Source: CAD feature listing. Evaluate the final solid. Frame: model axes, mm. A direction names the side the tool comes from. Give positions to 0.01 mm unless a question says otherwise; leave off trailing zeros. Order: outer loops, then holes, each group sorted by start corner. A loop starts at its lowest first (then second) coordinate and runs counter-clockwise, first axis right, second up. Notation, with made-up numbers: (52.25, 14.5) -> (92.25, 14.5) arc R12 ccw to (92.25, 25.5) -> close; hole circle Ø3 at (-29, 55). An arc over 180 degrees is marked (long way). Use CSV: the item, a comma, the result in double quotes.
```python
from build123d import *

# Parameters (mm, degrees)
F1_DEPTH = 2.286
F2_DEPTH = 0.254
F3_W     = 12.7
F3_H     = 1.016
F4_DEPTH = 0.254


with BuildPart() as f1:
    # F0 (on Top) → F1 (new body)
    with BuildSketch(Plane.XY):
        with BuildLine():
            Line((-13.1568801942, -7.1914618043), (-15.685681705, -13.4825458221))
            add(Edge.make_bspline(
                [(-15.685681705, -13.4825458221), (-13.2321975411, -12.2693498698), (-11.0318471059, -10.4379374373), (-8.9577929719, -8.5581073527)],
                knots=[0, 0, 0, 0, 6.5648699385, 6.5648699385, 6.5648699385, 6.5648699385], degree=3))
            add(Edge.make_bspline(
                [(-8.9577929719, -8.5581073527), (-2.326521087, -2.5478185256), (3.0136976356, 3.9574156183), (11.2083703228, -7.6654970922)],
                knots=[6.5648699385, 6.5648699385, 6.5648699385, 6.5648699385, 27.554407645, 27.554407645, 27.554407645, 27.554407645], degree=3))
            add(Edge.make_bspline(
                [(11.2083703228, -7.6654970922), (12.3264260334, -9.2512912326), (13.497617481, -11.1745413121), (14.7324733271, -13.4825458221)],
                knots=[27.554407645, 27.554407645, 27.554407645, 27.554407645, 30.4181550321, 30.4181550321, 30.4181550321, 30.4181550321], degree=3))
            Line((14.7324733271, -13.4825458221), (12.2638968299, -7.2552273315))
            Line((12.2638968299, -7.2552273315), (5.6394149783, 9.4559251776))
            Line((5.6394149783, 9.4559251776), (-0.3707793305, 24.6174541779))
            Line((-0.3707793305, 24.6174541779), (-6.4710147318, 9.441453502))
            Line((-6.4710147318, 9.441453502), (-13.1568801942, -7.1914618043))
        make_face()
        with BuildLine():
            add(Edge.make_bspline(
                [(-6.4710147318, 9.441453502), (-39.6247541981, 4.06906696), (-13.1568801942, -7.1914618043)],
                knots=[1.8867642182, 1.8867642182, 1.8867642182, 4.0030869743, 4.0030869743, 4.0030869743], degree=2, weights=[1, 0.4904751866, 1]))
            Line((-13.1568801942, -7.1914618043), (-6.4710147318, 9.441453502))
        make_face()
        with BuildLine():
            add(Edge.make_bspline(
                [(-8.9577929719, -8.5581073527), (-2.326521087, -2.5478185256), (3.0136976356, 3.9574156183), (11.2083703228, -7.6654970922)],
                knots=[6.5648699385, 6.5648699385, 6.5648699385, 6.5648699385, 27.554407645, 27.554407645, 27.554407645, 27.554407645], degree=3))
            add(Edge.make_bspline(
                [(-8.9577929719, -8.5581073527), (1.6671986102, -11.1197744869), (11.2083703228, -7.6654970922)],
                knots=[4.2596733084, 4.2596733084, 4.2596733084, 5.3432299115, 5.3432299115, 5.3432299115], degree=2, weights=[1, 0.8567930368, 1]))
        make_face()
        with BuildLine():
            add(Edge.make_bspline(
                [(12.2638968299, -7.2552273315), (39.4332818564, 4.06906696), (5.6394149783, 9.4559251776)],
                knots=[5.4115698154, 5.4115698154, 5.4115698154, 7.5428353935, 7.5428353935, 7.5428353935], degree=2, weights=[1, 0.4839505579, 1]))
            Line((5.6394149783, 9.4559251776), (12.2638968299, -7.2552273315))
        make_face()
    extrude(amount=-F1_DEPTH)

    # F0 (on Top) → F2 (cut)
    with BuildSketch(Plane.XY):
        with BuildLine():
            add(Edge.make_bspline(
                [(-6.4710147318, 9.441453502), (-39.6247541981, 4.06906696), (-13.1568801942, -7.1914618043)],
                knots=[1.8867642182, 1.8867642182, 1.8867642182, 4.0030869743, 4.0030869743, 4.0030869743], degree=2, weights=[1, 0.4904751866, 1]))
            Line((-13.1568801942, -7.1914618043), (-6.4710147318, 9.441453502))
        make_face()
        with BuildLine():
            add(Edge.make_bspline(
                [(12.2638968299, -7.2552273315), (39.4332818564, 4.06906696), (5.6394149783, 9.4559251776)],
                knots=[5.4115698154, 5.4115698154, 5.4115698154, 7.5428353935, 7.5428353935, 7.5428353935], degree=2, weights=[1, 0.4839505579, 1]))
            Line((5.6394149783, 9.4559251776), (12.2638968299, -7.2552273315))
        make_face()
        with BuildLine():
            add(Edge.make_bspline(
                [(-8.9577929719, -8.5581073527), (-2.326521087, -2.5478185256), (3.0136976356, 3.9574156183), (11.2083703228, -7.6654970922)],
                knots=[6.5648699385, 6.5648699385, 6.5648699385, 6.5648699385, 27.554407645, 27.554407645, 27.554407645, 27.554407645], degree=3))
            add(Edge.make_bspline(
                [(-8.9577929719, -8.5581073527), (1.6671986102, -11.1197744869), (11.2083703228, -7.6654970922)],
                knots=[4.2596733084, 4.2596733084, 4.2596733084, 5.3432299115, 5.3432299115, 5.3432299115], degree=2, weights=[1, 0.8567930368, 1]))
        make_face()
    extrude(amount=-F2_DEPTH, mode=Mode.SUBTRACT)

    # F3 (on face) → F4 (cut)
    with BuildSketch(Plane(origin=(0, 0, -2.286), x_dir=(1, 0, 0), z_dir=(0, 0, -1))):
        with Locations((0.1644820441, -1.469257871)):
            Rectangle(F3_W, F3_H)
    extrude(amount=-F4_DEPTH, mode=Mode.SUBTRACT)


solid = f1.part
```
1. Access query for faces 1 (the flat face through (-13, 2, -0.254)), 2 (the flat face through (12, 1, -0.254)), 3 (the flat face through (-2, 6, 0)). Directions: +Z, -Z, +X, -X, +Y, -Y. A direction counts if a zero-diameter tool reaches every point of the face in a straight line with its end or side. Return the directions, or none.
Answer below:
face 1,"+Z, -X, +Y"
face 2,"+Z, +X, +Y"
face 3,"+Z, +X, -X, +Y, -Y"
2. Ray query, line 1 along Z through (x, y) = (16.5, 2); line 2 along X through (y, z) = (21, -0.15); line 3 along Y through (x, z) = (-4.5, -2). Return the intervals inside material, ascending.
Answer below:
line 1,"z = -2.29 to -0.25"
line 2,"x = -1.82 to 1.06"
line 3,"y = -9.32 to 14.34"
3. Pin query (flat end, axial travel): P1, Ø6, axis at x = -9, y = 12.5, coming from the +Z side; P2, Ø2.5, axis at x = -3.5, y = -7.5, coming from the +Z side; P3, Ø1, axis at x = -10, z = -1, coming from the -Y side. Return the tip coordinate at first contact, or that it passes through.
Answer below:
P1,"passes through"
P2,"stops at z = -0.25"
P3,"stops at y = -9.92"
4. Section query A-A on y = 22. Return loops of the section in (x, z), plus the area to 3 significant figures.
Answer below:
outline,"(-1.42, -2.29) -> (0.67, -2.29) -> (0.67, 0) -> (-1.42, 0) -> close"
area,"4.78 mm²"
5. Mould query, pull axis Y, two halves, no side actions, for faces 4 (the flat face through (0.1, 1.5, -2.032)), 5 (the flat face through (2, -6, -0.254)). Classes: released by +Y, released by -Y, zero draft, split by the parting line, or undercut.
Answer below:
face 4,"undercut"
face 5,"zero draft"
